from build123d import *

# Parameters (mm, degrees)
SKETCH1_R           = 0.65
BOSS_EXTRUDE1_DEPTH = 1


with BuildPart() as part:
    # Sketch1 → Boss-Extrude1 (new body)
    with BuildSketch(Plane(origin=(0, 0, 0), x_dir=(1, 0, 0), z_dir=(0, 1, 0))):
        with BuildLine():
            Line((-0.5, -7.583534796), (-0.5, -5.477225575))
            ThreePointArc((-0.5, -5.477225575), (-1.148443874, -5.37876163), (-1.780556133, -5.203808207))
            ThreePointArc((-1.780556133, -5.203808207), (-3.318545169, -4.906574915), (-4.553408035, -3.94279506))
            ThreePointArc((-4.553408035, -3.94279506), (0, 5.5), (4.553408035, -3.94279506))
            ThreePointArc((4.553408035, -3.94279506), (3.318545169, -4.906574915), (1.780556133, -5.203808207))
            ThreePointArc((1.780556133, -5.203808207), (1.148443874, -5.37876163), (0.5, -5.477225575))
            Line((0.5, -5.477225575), (0.5, -7.583534796))
            ThreePointArc((0.5, -7.583534796), (0, 7.6), (-0.5, -7.583534796))
        make_face()
        with Locations(Location((-1.5, -6.329588857, 0), (0, 0, 270))):
            Circle(SKETCH1_R, mode=Mode.SUBTRACT)
        with Locations(Location((1.5, -6.329588857, 0), (0, 0, 90))):
            Circle(SKETCH1_R, mode=Mode.SUBTRACT)
    extrude(amount=BOSS_EXTRUDE1_DEPTH)


solid = part.part
Could you check a few things on this model? Use its own coordinates, in mm. A direction names the side the tool comes from. Coordinates: 2 decimals unless noted, no trailing zeros. Write each loop counter-clockwise with the first axis right and the second up, starting at its lowest first coordinate (ties: lowest second). Pieces come first, ordered by that corner, then holes. Notation, with made-up numbers: (73, 64.5) - (127, 64.5) arc R13 cw to (127, 73.5) - close; hole circle Ø4 at (36, 35). An arc over 180 degrees is marked (long way). Put each result on its own line as item: value. Start each with the question number.
Q1. Thinking about a two-plate mould opening in Z: for faces 4 (the cylindrical face through (0.327, 0.493, -7.593)), 5 (the cylindrical face through (-0.183, 0.493, -5.497)), 6 (the flat face through (-0.5, 0.5, 6.5)), 7 (the cylindrical face through (-1.14, 0.49, 5.38)), which applies, pulls with the +Z half, pulls with the -Z half, needs draft (parallel to the pull), parting line crosses it, or undercut?
Q2. I want a section at C-C on y = 0.55. Write out the boundary of the cut face in (x, z), plus the area to 3 significant figures.
Q3. Which directions (+Z, -Z, +X, -X, +Y, -Y) give clear straight access to the entire face, cutting with the end or side of a thin tool? Please do faces 1 (the flat face through (1.1, 1, 5.6)), 2 (the flat face through (0.5, 0.5, 6.5)), 3 (the cylindrical face through (3.339, 0.493, 4.897)).
Q4. I'm going to push flat-ended pins straight in: P1, Ø1.7, axis at x = 1.5, z = 6.33, coming from the +Y side; P2, Ø0.8, axis at x = -1.5, z = 6.33, coming from the -Y side. Where does each tip first touch, or does it pass through?
Q5. I want a section at A-A on x = 4.25. Write out the boundary of the cut face in (y, z).
Q6. I want a section at B-B on z = 0. Write out the boundary of the cut face in (x, y), plus the area to 3 significant figures.
Q7. I want a section at D-D on z = 6.25. Write out the boundary of the cut face in (x, y).
Q8. Please list where these lines run through material, in increasing order: L1, parallel to Z at x = -1.25, y = 0.95; L2, parallel to Z at x = -2, y = 0.7; L3, parallel to X at y = 0.5, z = 6.75.
Checks:
1. face 4: parting line crosses it
1. face 5: undercut
1. face 6: needs draft
1. face 7: undercut
2. outline: (-4.55, 3.94) arc R3.35 cw to (-1.78, 5.2) arc R5.5 cw to (-0.5, 5.48) - (-0.5, 7.58) arc R7.6 ccw (long way) to (0.5, 7.58) - (0.5, 5.48) arc R5.5 cw to (1.78, 5.2) arc R3.35 cw to (4.55, 3.94) arc R5.82 cw (long way) to start; hole circle Ø1.3 at (-1.5, 6.33); hole circle Ø1.3 at (1.5, 6.33)
2. area: 74.0 mm²
3. face 1: +Z, -Z, +X, -X, +Y
3. face 2: +Z, +Y, -Y
3. face 3: +Y, -Y
4. P1: y = 1
4. P2: through
5. outline: (0, -6.3) - (1, -6.3) - (1, -3.66) - (0, -3.66) - close; (0, 4.28) - (1, 4.28) - (1, 6.3) - (0, 6.3) - close
6. outline: (-7.6, 0) - (-5.81, 0) - (-5.81, 1) - (-7.6, 1) - close; (5.81, 0) - (7.6, 0) - (7.6, 1) - (5.81, 1) - close
6. area: 3.58 mm²
7. outline: (-4.32, 0) - (-2.15, 0) - (-2.15, 1) - (-4.32, 1) - close; (-0.85, 0) - (-0.5, 0) - (-0.5, 1) - (-0.85, 1) - close; (0.5, 0) - (0.85, 0) - (0.85, 1) - (0.5, 1) - close; (2.15, 0) - (4.32, 0) - (4.32, 1) - (2.15, 1) - close
8. L1: -7.5 to -5.36, 5.36 to 5.73, 6.93 to 7.5
8. L2: -7.33 to -5.15, 5.21 to 5.91, 6.74 to 7.33
8. L3: -3.49 to -2, -1 to -0.5, 0.5 to 1, 2 to 3.49
